from build123d import *

# Parameters (mm, degrees)
F1_DEPTH = 25
F3_W     = 7
F3_H     = 20.8
F4_DEPTH = 10
F5_R     = 1.25
F6_DEPTH = 25
F7_R     = 4
F8_R     = 8


with BuildPart() as f1:
    # F0 (on Top) → F1 (new body)
    with BuildSketch(Plane.XY):
        Polygon((0, 20), (0, 0), (9.1, 0), (9.1, 2.1), (2.1, 2.1), (2.1, 22.1), (-15.1, 22.1), (-15.1, 2.1), (-23, 2.1), (-23, 0), (-13, 0), (-13, 20), align=None)
        Polygon((9.1, 2.1), (9.1, 0), (19.1419273615, 0), (19.1419273615, 8.9497342706), (9.1, 8.9497342706), align=None)
    extrude(amount=F1_DEPTH)

    # F3 (on offset) → F4 (cut)
    with BuildSketch(Plane.YZ.offset(19.1419273615)):
        with Locations((3.5, 12.5)):
            Rectangle(F3_W, F3_H)
    extrude(amount=-F4_DEPTH, mode=Mode.SUBTRACT)

    # F5 (on Front) → F6 (cut)
    with BuildSketch(Plane.XZ):
        with Locations((-19, 12.5)):
            Circle(F5_R)
        with Locations((5.5, 12.5)):
            Circle(F5_R)
    extrude(amount=-F6_DEPTH, mode=Mode.SUBTRACT)

    # F7
    f7_edges = [f1.edges().sort_by_distance(p)[0] for p in [
        (-15.1, 22.1, 12.5),
        (2.1, 22.1, 12.5),
        (14.120964, 8.949734, 25),
        (14.120964, 8.949734, 0),
        (-23, 1.05, 25),
        (-23, 1.05, 0),
        (19.141927, 4.474867, 25),
        (19.141927, 4.474867, 0),
    ]]
    fillet(f7_edges, radius=F7_R)

    # F8
    f8_edges = [f1.edges().sort_by_distance(p)[0] for p in [
        (9.141927, 3.5, 22.9),
    ]]
    fillet(f8_edges, radius=F8_R)


solid = f1.part
Check sheet for the modelled part. Datum: model origin and axes. Units: mm. A direction names the side the tool comes from. Round coordinates to 2 decimals unless told otherwise and drop trailing zeros. Loops run counter-clockwise (first coordinate to the right, second up) from the corner with the lowest first, then second, coordinate; pieces in that order, holes last.
1. Gauge pin test, flat ends, axial feed: pin 1 Ø5 at (x, z) = (3.5, 19) entering from +Y (3 decimals); pin 2 Ø6.5 at (x, z) = (-3.5, 13.5) entering from -Y; pin 3 Ø3.5 at (y, z) = (3.5, 7.5) entering from +X; pin 4 Ø2 at (x, z) = (-19, 12.5) entering from -Y. Record the tip position at first contact, or that the pin passes through.
2. Sectioned sample at A-A on z = 12.5. Record the boundary of the cut face in (x, y), and give its area (3 significant figures).
3. Sectioned sample at D-D on z = 6. Record the boundary of the cut face in (x, y), and give its area (3 significant figures).
4. Scan lines: probe 1 along X at (y, z) = (8.25, 14.5); probe 2 along Z at (x, y) = (5.5, 0.75); probe 3 along X at (y, z) = (5.25, 20.5). Record each from-to range of solid material in increasing order.
5. Set-up check for faces 4 (the flat face through (14, 8.95, 12)), 5 (the flat face through (18, 3, 22.9)), 6 (the flat face through (2.1, 10, 12)), 7 (the flat face through (-17, 2.1, 12)): record each of +Z, -Z, +X, -X, +Y, -Y from which the full face is reachable in a straight line by a thin tool's end or side.
6. Sectioned sample at C-C on y = 11. Record the boundary of the cut face in (x, z).
7. Sectioned sample at B-B on x = 5.5. Record the boundary of the cut face in (y, z), and give its area (4 significant figures).
8. Mould release check, pull along Z, two halves, no side actions. Record for faces 1 (the flat face through (1, 9, 25)), 2 (the flat face through (14, 7, 12)), 3 (the cylindrical face through (17.4, 4.5, 0.7)): released by +Z, released by -Z, zero draft, split by the parting line, or undercut.
Recorded:
1. pin 1: stops at y = 20.855
1. pin 2: stops at y = 20
1. pin 3: stops at x = 9.14
1. pin 4: passes through
2. outline: (-23, 0) - (-20.25, 0) - (-20.25, 2.1) - (-23, 2.1) - close; (-17.75, 0) - (-13, 0) - (-13, 20) - (0, 20) - (0, 0) - (4.25, 0) - (4.25, 2.1) - (2.1, 2.1) - (2.1, 18.1) arc R4 ccw to (-1.9, 22.1) - (-11.1, 22.1) arc R4 ccw to (-15.1, 18.1) - (-15.1, 2.1) - (-17.75, 2.1) - close; (6.75, 0) - (9.14, 0) - (9.14, 7) - (19.14, 7) - (19.14, 8.95) - (9.1, 8.95) - (9.1, 2.1) - (6.75, 2.1) - close
2. area: 154 mm2
3. outline: (-23, 0) - (-13, 0) - (-13, 20) - (0, 20) - (0, 0) - (9.14, 0) - (9.14, 7) - (19.14, 7) - (19.14, 8.95) - (9.1, 8.95) - (9.1, 2.1) - (2.1, 2.1) - (2.1, 18.1) arc R4 ccw to (-1.9, 22.1) - (-11.1, 22.1) arc R4 ccw to (-15.1, 18.1) - (-15.1, 2.1) - (-23, 2.1) - close
3. area: 164 mm2
4. probe 1: x = -15.1 to -13, 0 to 2.1, 9.1 to 19.14
4. probe 2: z = 0 to 11.25, 13.75 to 25
4. probe 3: x = -15.1 to -13, 0 to 2.1, 9.1 to 11.43
5. face 4: +Z, -Z, +X, +Y
5. face 5: +X, -Y
5. face 6: +Z, -Z, +Y
5. face 7: +Z, -Z, -X, +Y
6. outline: (-15.1, 0) - (-13, 0) - (-13, 25) - (-15.1, 25) - close; (0, 0) - (2.1, 0) - (2.1, 25) - (0, 25) - close
7. outline: (0, 0) - (2.1, 0) - (2.1, 11.25) - (0, 11.25) - close; (0, 13.75) - (2.1, 13.75) - (2.1, 25) - (0, 25) - close
7. area: 47.25 mm2
8. face 1: released by +Z
8. face 2: undercut
8. face 3: released by -Z
